The model under review builds one solid part; all positions refer to its coordinate system, in mm. Face numbers are marked on the shaded views. A direction names the side the tool comes from. Coordinates: 2 decimals unless noted, no trailing zeros. Loops run counter-clockwise (first coordinate to the right, second up) from the corner with the lowest first, then second, coordinate; pieces in that order, holes last. Notation, with made-up numbers: M 23,36.5 L 47,36.5 A9 cw 47,48.5 Z; hole C 68.25,-9.75 d7. An arc over 180 degrees is marked long. Use CSV: the item, a comma, the result in double quotes. Start each with the question number.
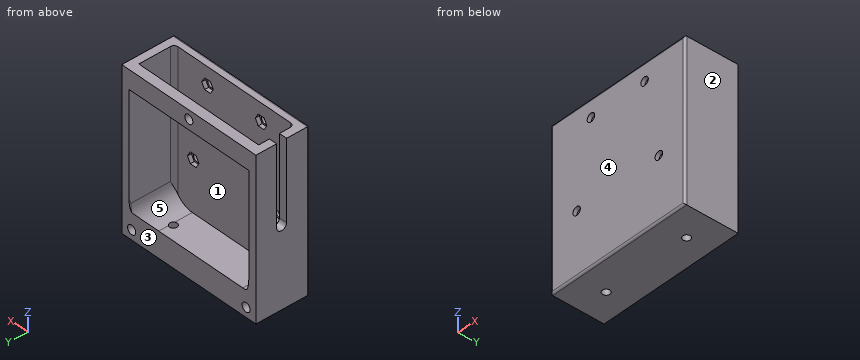
from build123d import *

# Parameters (mm, degrees)
EXTRUDE_1_DEPTH          = 37.5
SHELL_START              = -33.5
SHELL_1_DEPTH            = 67
FILLET_1_R               = 5
FILLET_3_R               = 2
FILLET_4_R               = 1
FILLET_5_R               = 10
CUT_EXTRUDE_2_DEPTH      = 94.307288118
CUT_EXTRUDE_2_DEPTH_BACK = 3
SKETCH_3_R               = 1.9
CUT_EXTRUDE_1_DEPTH      = 103.419810279
CUT_EXTRUDE_1_DEPTH_BACK = 103.419810279
SKETCH_2_W               = 80
SKETCH_2_H               = 35
SKETCH_5_R               = 2.25
CUT_EXTRUDE_4_DEPTH      = 8
CUT_EXTRUDE_5_DEPTH      = 88.242478302
CUT_EXTRUDE_5_DEPTH_BACK = 88.242478302
SKETCH_6_R               = 1.9
CUT_EXTRUDE_6_REACH      = 114.934
CUT_EXTRUDE_7_REACH      = 94.386
SKETCH_8_R               = 2.1
CUT_EXTRUDE_8_DEPTH      = 2


# Read off the part's stored shape, not the designer's step: 抽壳1
with BuildPart() as part:
    # 草图1 → 凸台-拉伸1 (new, symmetric)
    with BuildSketch(Plane(origin=(0, 0, 0), x_dir=(0, 0, -1), z_dir=(1, 0, 0))):
        Polygon((-70.540010176, 52.231309316), (-70.540010176, 30), (-80, 30), (-80, 0), (0, 0), (0, 30), (-9.459989824, 30), align=None)
    extrude(amount=EXTRUDE_1_DEPTH, both=True)

    # 抽壳1 outline → 抽壳1 (cut)
    with BuildSketch(Plane.YZ.offset(SHELL_START)):
        Polygon((47.974598226, 70.540010176), (22, 70.540010176), (22, 80), (4, 80), (4, 6), (24.483955603, 6), align=None)
    extrude(amount=SHELL_1_DEPTH, mode=Mode.SUBTRACT)

    # 圆角1
    fillet_1_edges = [part.edges().sort_by_distance(p)[0] for p in [
        (0, 30, 9.459989824),
        (35.5, 30, 70.540010176),
        (-35.5, 30, 70.540010176),
    ]]
    fillet(fillet_1_edges, radius=FILLET_1_R)

    # 圆角3
    fillet_3_edges = [part.edges().sort_by_distance(p)[0] for p in [
        (33.5, 4, 43),
        (33.5, 36.229276914, 38.270005088),
        (-33.5, 36.229276914, 38.270005088),
        (-33.5, 4, 43),
    ]]
    fillet(fillet_3_edges, radius=FILLET_3_R)

    # 圆角4
    fillet_4_edges = [part.edges().sort_by_distance(p)[0] for p in [
        (-37.5, 30, 4.28917746),
        (-37.5, 30.075961235, 9.446595809),
        (37.5, 30, 4.28917746),
        (37.5, 30.075961235, 9.446595809),
        (-37.5, 41.266423106, 40.414232907),
        (0, 52.231309316, 70.540010176),
        (37.5, 41.266423106, 40.414232907),
        (37.5, 0, 40),
        (-37.5, 0, 40),
        (0, 0, 80),
        (0, 0, 0),
        (0, 30, 0),
        (0, 30, 80),
    ]]
    fillet(fillet_4_edges, radius=FILLET_4_R)

    # 圆角5
    # the kernel refuses this fillet: 10 mm, written as the material it adds along each edge
    with BuildSketch(Plane(origin=(33.5, -19, 6), x_dir=(0, 0, 1), z_dir=(0, 1, 0))) as fillet_5_piece_1_section:
        with BuildLine():
            CenterArc((FILLET_5_R, -FILLET_5_R), FILLET_5_R, 90, 90)
            Line((0, -FILLET_5_R), (0, 0))
            Line((0, 0), (FILLET_5_R, 0))
        make_face()
    fillet_5_piece_1 = extrude(amount=66.355600058, mode=Mode.PRIVATE)
    fillet_5_piece_1 = split(fillet_5_piece_1, bisect_by=Plane(origin=(31.283756862, 30, 8.259643185), z_dir=(0, -1, 0)), keep=Keep.TOP, mode=Mode.PRIVATE)
    fillet_5_piece_1 = split(fillet_5_piece_1, bisect_by=Plane(origin=(31.283756862, 0, 8.259643185), z_dir=(0, 1, 0)), keep=Keep.TOP, mode=Mode.PRIVATE)
    add(fillet_5_piece_1)
    with BuildSketch(Plane(origin=(-33.5, -19, 6), x_dir=(0, 0, 1), z_dir=(0, 1, 0))) as fillet_5_piece_2_section:
        with BuildLine():
            CenterArc((FILLET_5_R, FILLET_5_R), FILLET_5_R, 180, 90)
            Line((0, FILLET_5_R), (0, 0))
            Line((0, 0), (FILLET_5_R, 0))
        make_face()
    fillet_5_piece_2 = extrude(amount=66.355600058, mode=Mode.PRIVATE)
    fillet_5_piece_2 = split(fillet_5_piece_2, bisect_by=Plane(origin=(-31.283756862, 30, 8.259643185), z_dir=(0, -1, 0)), keep=Keep.TOP, mode=Mode.PRIVATE)
    fillet_5_piece_2 = split(fillet_5_piece_2, bisect_by=Plane(origin=(-31.283756862, 0, 8.259643185), z_dir=(0, 1, 0)), keep=Keep.TOP, mode=Mode.PRIVATE)
    add(fillet_5_piece_2)

    # 草图3 → 切除-拉伸2 (cut, two sides: drawn at the far end of the back side and taken through both)
    with BuildSketch(Plane(origin=(0, 30, 0), x_dir=(1, 0, 0), z_dir=(0, 1, 0)).offset(-CUT_EXTRUDE_2_DEPTH_BACK)):
        with Locations(Location((-32, -4.78917746, 0), (0, 0, 90))):
            Circle(SKETCH_3_R)
        with Locations(Location((32, -4.78917746, 0), (0, 0, 90))):
            Circle(SKETCH_3_R)
        with Locations(Location((0, -75.540010176, 0), (0, 0, 90))):
            Circle(SKETCH_3_R)
    extrude(amount=CUT_EXTRUDE_2_DEPTH + CUT_EXTRUDE_2_DEPTH_BACK, mode=Mode.SUBTRACT)

    # 草图2 → 切除-拉伸1 (cut, two sides: drawn at the far end of the back side and taken through both)
    with BuildSketch(Plane(origin=(0, 0, 0), x_dir=(0, 0, -1), z_dir=(1, 0, 0)).offset(-CUT_EXTRUDE_1_DEPTH_BACK)):
        with Locations((-40, 44.5)):
            Rectangle(SKETCH_2_W, SKETCH_2_H)
    extrude(amount=CUT_EXTRUDE_1_DEPTH + CUT_EXTRUDE_1_DEPTH_BACK, mode=Mode.SUBTRACT)

    # 草图5 → 切除-拉伸4 (cut)
    with BuildSketch(Plane(origin=(0, 27, 0), x_dir=(1, 0, 0), z_dir=(0, 1, 0))):
        with Locations(Location((0, -75.540010176, 0), (0, 0, 270))):
            Circle(SKETCH_5_R)
        with Locations(Location((32, -4.78917746, 0), (0, 0, 270))):
            Circle(SKETCH_5_R)
        with Locations(Location((-32, -4.78917746, 0), (0, 0, 270))):
            Circle(SKETCH_5_R)
    extrude(amount=-CUT_EXTRUDE_4_DEPTH, mode=Mode.SUBTRACT)

    # 草图6 → 切除-拉伸5 (cut, two sides: drawn at the far end of the back side and taken through both)
    with BuildSketch(Plane.XY.offset(6).offset(-CUT_EXTRUDE_5_DEPTH_BACK)):
        with Locations((-22.5, 14.5)):
            Circle(SKETCH_6_R)
        with Locations((22.5, 14.5)):
            Circle(SKETCH_6_R)
    extrude(amount=CUT_EXTRUDE_5_DEPTH + CUT_EXTRUDE_5_DEPTH_BACK, mode=Mode.SUBTRACT)

    # 草图7 → 切除-拉伸6 (cut, up to next)
    with BuildSketch(Plane.ZY.offset(37.5), mode=Mode.PRIVATE) as cut_extrude_6_sk1:
        with BuildLine():
            Line((40, 16.5), (80, 16.5))
            ThreePointArc((80, 16.5), (82.5, 14), (80, 11.5))
            Line((80, 11.5), (40, 11.5))
            ThreePointArc((40, 11.5), (37.5, 14), (40, 16.5))
        make_face()
    cut_extrude_6_tool1 = extrude(cut_extrude_6_sk1.sketch, amount=-CUT_EXTRUDE_6_REACH, mode=Mode.PRIVATE) & part.part
    add(cut_extrude_6_tool1.solids().sort_by_distance((-37.5, 14, 60))[0], mode=Mode.SUBTRACT)

    # 草图8 → 切除-拉伸7 (cut, up to next)
    with BuildSketch(Plane.XZ, mode=Mode.PRIVATE) as cut_extrude_7_sk1:
        with Locations(Location((23, 31.28, 0), (0, 0, 270))):
            Circle(SKETCH_8_R)
    cut_extrude_7_tool1 = extrude(cut_extrude_7_sk1.sketch, amount=-CUT_EXTRUDE_7_REACH, mode=Mode.PRIVATE) & part.part
    # 草图8 → 切除-拉伸7 (cut, up to next)
    with BuildSketch(Plane.XZ, mode=Mode.PRIVATE) as cut_extrude_7_sk2:
        with Locations(Location((15, 71, 0), (0, 0, 270))):
            Circle(SKETCH_8_R)
    cut_extrude_7_tool2 = extrude(cut_extrude_7_sk2.sketch, amount=-CUT_EXTRUDE_7_REACH, mode=Mode.PRIVATE) & part.part
    # 草图8 → 切除-拉伸7 (cut, up to next)
    with BuildSketch(Plane.XZ, mode=Mode.PRIVATE) as cut_extrude_7_sk3:
        with Locations(Location((-15, 71, 0), (0, 0, 270))):
            Circle(SKETCH_8_R)
    cut_extrude_7_tool3 = extrude(cut_extrude_7_sk3.sketch, amount=-CUT_EXTRUDE_7_REACH, mode=Mode.PRIVATE) & part.part
    # 草图8 → 切除-拉伸7 (cut, up to next)
    with BuildSketch(Plane.XZ, mode=Mode.PRIVATE) as cut_extrude_7_sk4:
        with Locations(Location((-23, 31.28, 0), (0, 0, 270))):
            Circle(SKETCH_8_R)
    cut_extrude_7_tool4 = extrude(cut_extrude_7_sk4.sketch, amount=-CUT_EXTRUDE_7_REACH, mode=Mode.PRIVATE) & part.part
    add(cut_extrude_7_tool1.solids().sort_by_distance((23, 0, 31.28))[0], mode=Mode.SUBTRACT)
    add(cut_extrude_7_tool2.solids().sort_by_distance((15, 0, 71))[0], mode=Mode.SUBTRACT)
    add(cut_extrude_7_tool3.solids().sort_by_distance((-15, 0, 71))[0], mode=Mode.SUBTRACT)
    add(cut_extrude_7_tool4.solids().sort_by_distance((-23, 0, 31.28))[0], mode=Mode.SUBTRACT)

    # 草图9 → 切除-拉伸8 (cut)
    with BuildSketch(Plane(origin=(0, 4, 0), x_dir=(1, 0, 0), z_dir=(0, 1, 0))):
        Polygon((18.233161507, -71), (16.616580754, -68.2), (13.383419246, -68.2), (11.766838493, -71), (13.383419246, -73.8), (16.616580754, -73.8), align=None)
        Polygon((-11.766838493, -71), (-13.383419246, -68.2), (-16.616580754, -68.2), (-18.233161507, -71), (-16.616580754, -73.8), (-13.383419246, -73.8), align=None)
        Polygon((26.233161507, -31.28), (24.616580754, -28.48), (21.383419246, -28.48), (19.766838493, -31.28), (21.383419246, -34.08), (24.616580754, -34.08), align=None)
        Polygon((-26.233161507, -31.28), (-24.616580754, -34.08), (-21.383419246, -34.08), (-19.766838493, -31.28), (-21.383419246, -28.48), (-24.616580754, -28.48), align=None)
    extrude(amount=-CUT_EXTRUDE_8_DEPTH, mode=Mode.SUBTRACT)


solid = part.part
1. Draft analysis for pull direction Y (two halves, no side actions). For the marked faces 3, 4 and 5, state which applies: released by +Y, released by -Y, zero draft, split by the parting line, or undercut.
2. Add section A-A (z = 41). Write out the cut boundary in (x, y).
3. Insertion check: pin 1 Ø5 at (x, z) = (23, 31.28) entering from +Y; pin 2 Ø8 at (x, z) = (-15.5, 32.5) entering from +Y; pin 3 Ø1 at (x, y) = (15.5, 3) entering from -Z; pin 4 Ø3 at (x, y) = (9, 8.5) entering from +Z. Each pin has a flat end and moves straight along its axis. Give the tip position at first contact, or say it passes through.
4. Add section D-D (y = 23.25). Write out the cut boundary in (x, z), plus the area to 3 significant figures.
5. For the marked faces 1 and 2, list the 3-axis set-ups (+Z, -Z, +X, -X, +Y, -Y) from which the entire face can be reached by the end or side of a thin tool; tool diameter is ignored.
6. Add section B-B (x = -15). Write out the cut boundary in (y, z), plus the area to 3 significant figures.
7. To check wall thickness, follow line 1 along X through (y, z) = (1.2, 31.28); line 2 along X through (y, z) = (0.85, 71); line 3 along X through (y, z) = (9.75, 41). State the ranges of each line that lie inside material, in increasing order.
8. Add section C-C (x = -4.5). Write out the cut boundary in (y, z).
Solved:
1,face 3,"released by +Y"
1,face 4,"released by -Y"
1,face 5,"undercut"
2,outline,"M -37.5,1 A1 ccw -36.5,0 L 36.5,0 A1 ccw 37.5,1 L 37.5,27 L 33.5,27 L 33.5,6 A2 cw 31.5,4 L -31.5,4 A2 cw -33.5,6 L -33.5,11.5 L -37.5,11.5 Z; M -37.5,16.5 L -33.5,16.5 L -33.5,27 L -37.5,27 Z"
3,pin 1,"stops at y = 2"
3,pin 2,"stops at y = 4"
3,pin 3,"stops at z = 0"
3,pin 4,"stops at z = 6"
4,outline,"M -37.5,0 L 37.5,0 L 37.5,80 L -37.5,80 Z; hole C -32,4.79 d4.5; hole M -33.5,16 A10 ccw -23.5,6 L 23.5,6 A10 ccw 33.5,16 L 33.5,70.54 L -33.5,70.54 Z; hole C 0,75.54 d4.5; hole C 32,4.79 d4.5"
4,area,"1,670 mm^2"
5,face 1,"+Z"
5,face 2,"+Z, -Z, +X, +Y, -Y"
6,outline,"M 0,1 A1 ccw 1,0 L 27,0 L 27,12.91 L 24.48,6 L 4,6 L 4,68.2 L 2,68.2 L 2,68.9 L 0,68.9 Z; M 0,73.1 L 2,73.1 L 2,73.8 L 4,73.8 L 4,80 L 1,80 A1 ccw 0,79 Z; M 22,70.54 L 27,70.54 L 27,80 L 22,80 Z"
6,area,"494 mm^2"
7,line 1,"x = -37.5 to -25.1, -20.9 to 20.9, 25.1 to 37.5"
7,line 2,"x = -37.49 to -17.1, -12.9 to 12.9, 17.1 to 37.49"
7,line 3,"x = -37.5 to -33.5, 33.5 to 37.5"
8,outline,"M 0,1 A1 ccw 1,0 L 27,0 L 27,12.91 L 24.48,6 L 4,6 L 4,80 L 1,80 A1 ccw 0,79 Z; M 22,70.54 L 27,70.54 L 27,80 L 22,80 Z"
